Here's how the part is built. I have some questions about the finished solid (model axes, mm). A direction names the side the tool comes from. Round coordinates to 2 decimals unless told otherwise and drop trailing zeros. Loops run counter-clockwise (first coordinate to the right, second up) from the corner with the lowest first, then second, coordinate; pieces in that order, holes last. Notation, with made-up numbers: (-23.5, 60.25) - (-5.5, 60.25) arc R21 cw to (-5.5, 78.25) - close; hole circle Ø2 at (75.25, 50.5). An arc over 180 degrees is marked (long way). Answer as a JSON object with one key per item and string values. Group by question number.
1) If I drill on line 1 along Y through (x, z) = (68, 4.5); line 2 along X through (y, z) = (29, 6.75); line 3 along Y through (x, z) = (9.5, 0.8), over which ranges is the centre line in solid material (lowest first)? Write a range as [from, to].
2) I want a section at B-B, the plane x = 78.5. Please give me the cut outline in (y, z).
3) Which directions (+Z, -Z, +X, -X, +Y, -Y) give clear straight access to the entire face, cutting with the end or side of a thin tool? Please do faces 5 (the face through (44, 2, 6)), 6 (the face through (71.5, 3, 6)), 7 (the face through (37, 79, 6)), 8 (the face through (9, 73, 0)).
4) I want a section at A-A, the plane y = 73. Please give me the cut outline in (x, z).
5) If we mould it in two halves opening along X, with no side actions, what happens to faces 1 (the face through (44, 80, 6)), 2 (the face through (0.57, 0.6, 0.85)), 3 (the face through (89, 42, 1)), 4 (the face through (23, 81, 2.6))? For each: pulls with the +X half, pulls with the -X half, needs draft (parallel to the pull), parting line crosses it, or undercut.
6) I want a section at D-D, the plane x = 26. Please give me the cut outline in (y, z), then the cut area to 3 significant figures.
7) I want a section at C-C, the plane y = 50. Please give me the cut outline in (x, z), then the cut area to 3 significant figures.
8) Will these pins go through, and if not, where does the flat tip stop? P1, Ø0.6, axis at y = 79, z = 6, coming from the +X side; P2, Ø1.6, axis at x = 13, y = 20, coming from the +Z side; P3, Ø1, axis at y = 81, z = 3, coming from the +X side.
from build123d import *

# Parameters (mm, degrees)
SKETCH_W        = 89
SKETCH_H        = 82
SKETCH_W_2      = 81
SKETCH_H_2      = 74
PAD_DEPTH       = 4.6
SKETCH001_W     = 89
SKETCH001_H     = 82
PAD001_DEPTH    = 3
SKETCH002_R     = 2.75
SKETCH002_R_2   = 1.25
PAD002_DEPTH    = 3
SKETCH003_W     = 15
SKETCH003_H     = 15
PAD003_DEPTH    = 3
FILLET_R        = 2
CHAMFER_SIZE    = 0.3
SKETCH004_W     = 15
SKETCH004_H     = 2
SKETCH004_W_2   = 54
SKETCH004_H_2   = 2.0000000001
PAD004_DEPTH    = 3
CHAMFER001_SIZE = 0.707
SKETCH010_W     = 12
SKETCH010_H     = 2
POCKET003_DEPTH = 2


with BuildPart() as part:
    # Sketch → Pad (new body)
    with BuildSketch(Plane.XY):
        with Locations((44.5, 41)):
            Rectangle(SKETCH_W, SKETCH_H)
        with Locations((44.5, 41)):
            Rectangle(SKETCH_W_2, SKETCH_H_2, mode=Mode.SUBTRACT)
    extrude(amount=PAD_DEPTH)

    # Sketch001 (on Face9 of Pad) → Pad001 (join)
    with BuildSketch(Plane(origin=(0, 0, 0), x_dir=(1, 0, 0), z_dir=(0, 0, -1))):
        with Locations((44.5, -41)):
            Rectangle(SKETCH001_W, SKETCH001_H)
    extrude(amount=PAD001_DEPTH)

    # Sketch002 (on Face8 of Pad001) → Pad002 (join)
    with BuildSketch(Plane.XY):
        with Locations((9.5, 73)):
            Circle(SKETCH002_R)
        with Locations((9.5, 73)):
            Circle(SKETCH002_R_2, mode=Mode.SUBTRACT)
        with Locations((78.5, 21)):
            Circle(SKETCH002_R)
        with Locations((78.5, 21)):
            Circle(SKETCH002_R_2, mode=Mode.SUBTRACT)
        with Locations((11.5, 21)):
            Circle(SKETCH002_R)
        with Locations((11.5, 21)):
            Circle(SKETCH002_R_2, mode=Mode.SUBTRACT)
    extrude(amount=PAD002_DEPTH)

    # Sketch003 (on Face11 of Pad002) → Pad003 (join)
    with BuildSketch(Plane.XY):
        with Locations((77.5, 70.5)):
            Rectangle(SKETCH003_W, SKETCH003_H)
    extrude(amount=PAD003_DEPTH)

    # Fillet
    fillet_edges = [part.edges().sort_by_distance(p)[0] for p in [
        (89, 0, 0.8),
        (89, 82, 0.8),
        (0, 0, 0.8),
        (0, 82, 0.8),
    ]]
    fillet(fillet_edges, radius=FILLET_R)

    # Chamfer
    chamfer_edges = [part.edges().sort_by_distance(p)[0] for p in [
        (8.25, 73, 3),
        (10.25, 21, 3),
        (77.25, 21, 3),
    ]]
    chamfer(chamfer_edges, length=CHAMFER_SIZE)

    # Sketch004 (on Face16 of Chamfer) → Pad004 (join)
    with BuildSketch(Plane.XY.offset(4.6)):
        Polygon((4, 78), (4, 4), (7.5, 4), (7.5, 1.9999999999), (2, 1.9999999999), (2, 80), (14, 80), (14, 78), align=None)
        Polygon((85, 4), (85, 78), (75, 78), (75, 80), (87, 80), (87, 1.9999999999), (81.5, 1.9999999999), (81.5, 4), align=None)
        with Locations((44.5, 79)):
            Rectangle(SKETCH004_W, SKETCH004_H)
        with Locations((44.5, 3)):
            Rectangle(SKETCH004_W_2, SKETCH004_H_2)
    extrude(amount=PAD004_DEPTH)

    # Chamfer001
    chamfer001_edges = [part.edges().sort_by_distance(p)[0] for p in [
        (8, 80, 7.6),
        (2, 41, 7.6),
        (44.5, 80, 7.6),
        (81, 80, 7.6),
        (87, 41, 7.6),
        (84.25, 2, 7.6),
        (44.5, 2, 7.6),
        (4.75, 2, 7.6),
    ]]
    chamfer(chamfer001_edges, length=CHAMFER001_SIZE)

    # Sketch010 (on Face16 of Chamfer001) → Pocket003 (cut)
    with BuildSketch(Plane(origin=(0, 82, 0), x_dir=(-1, 0, 0), z_dir=(0, 1, 0))):
        with Locations((-23.275, 3.6)):
            Rectangle(SKETCH010_W, SKETCH010_H)
    extrude(amount=-POCKET003_DEPTH, mode=Mode.SUBTRACT)


solid = part.part
Outcome:
{
 "1": {"line 1": "[0, 4], [78, 82]", "line 2": "[2, 4], [85, 87]", "line 3": "[0, 4], [19.11, 22.89], [70.25, 71.75], [74.25, 75.75], [78, 82]"},
 "2": {"outline": "(0, -3) - (82, -3) - (82, 4.6) - (80, 4.6) - (80, 6.89) - (79.29, 7.6) - (78, 7.6) - (78, 3) - (63, 3) - (63, 0) - (23.75, 0) - (23.75, 3) - (22.55, 3) - (22.25, 2.7) - (22.25, 0) - (19.75, 0) - (19.75, 2.7) - (19.45, 3) - (18.25, 3) - (18.25, 0) - (4, 0) - (4, 4.6) - (0, 4.6) - close"},
 "3": {"face 5": "+Z, +X, -X, -Y", "face 6": "+Z, +Y, -Y", "face 7": "+Z, +Y", "face 8": "+Z"},
 "4": {"outline": "(0, -3) - (89, -3) - (89, 4.6) - (87, 4.6) - (87, 6.89) - (86.29, 7.6) - (85, 7.6) - (85, 3) - (70, 3) - (70, 0) - (12.25, 0) - (12.25, 3) - (11.05, 3) - (10.75, 2.7) - (10.75, 0) - (8.25, 0) - (8.25, 2.7) - (7.95, 3) - (6.75, 3) - (6.75, 0) - (4, 0) - (4, 7.6) - (2.71, 7.6) - (2, 6.89) - (2, 4.6) - (0, 4.6) - close"},
 "5": {"face 1": "needs draft", "face 2": "pulls with the -X half", "face 3": "pulls with the +X half", "face 4": "undercut"},
 "6": {"outline": "(0, -3) - (82, -3) - (82, 2.6) - (80, 2.6) - (80, 4.6) - (78, 4.6) - (78, 0) - (4, 0) - (4, 7.6) - (2.71, 7.6) - (2, 6.89) - (2, 4.6) - (0, 4.6) - close", "area": "285 mm^2"},
 "7": {"outline": "(0, -3) - (89, -3) - (89, 4.6) - (87, 4.6) - (87, 6.89) - (86.29, 7.6) - (85, 7.6) - (85, 0) - (4, 0) - (4, 7.6) - (2.71, 7.6) - (2, 6.89) - (2, 4.6) - (0, 4.6) - close", "area": "315 mm^2"},
 "8": {"P1": "x = 87", "P2": "z = 3", "P3": "x = 88.94"}
}
